Print and shaded views of the part. All mm, measured from the part's lowest x, y and z. Give positions to 0.01 mm unless a question says otherwise; leave off trailing zeros. Order: outer loops, then holes, each group sorted by start corner. A loop starts at its lowest first (then second) coordinate and runs counter-clockwise, first axis right, second up. Notation, with made-up numbers: (-4.75, -8) -> (13.25, -8) arc R17 cw to (13.25, 18) -> close; hole circle Ø7 at (68, -10). An arc over 180 degrees is marked (long way). One line per question, with ' | ' between items. Start each with the question number.
(1) Cut at A-A (z = 19.05). Give the cut face in (x, y), then the cut area to 3 significant figures.
(2) Drill centre lines: L1, parallel to X at y = 9.25, z = 31.75; L2, parallel to X at y = 1.75, z = 42.5; L3, parallel to Z at x = 45.72, y = 3. Where is each one in solid material? Low to high. Write a range as from..to.
(3) Cut at B-B (y = 6.5). Give the number of separate pieces and of enclosed holes in the cut face, then the cut area to 3 significant figures.
(4) Cut at C-C (x = 71.12). Give the cut face in (y, z), then the cut area to 3 significant figures.
(5) Pin check, flat tips, straight feed: pin 1 Ø2 at (y, z) = (9.5, 40) entering from -X; pin 2 Ø4 at (x, z) = (45.72, 31.75) entering from -Y; pin 3 Ø3 at (x, y) = (14.5, 2.5) entering from +Z; pin 4 Ø3 at (x, y) = (21, 4) entering from -Z. Stop position of each tip, or through.
(6) Cut at D-D (x = 13). Give the cut face in (y, z) (1 decimal).
(7) Pull direction X, two halves, no side cores. Call the marked faces 1, 2, 3 and 4: +X half, -X half, draft (parallel to the pull), parting line (faces both ways), or undercut.
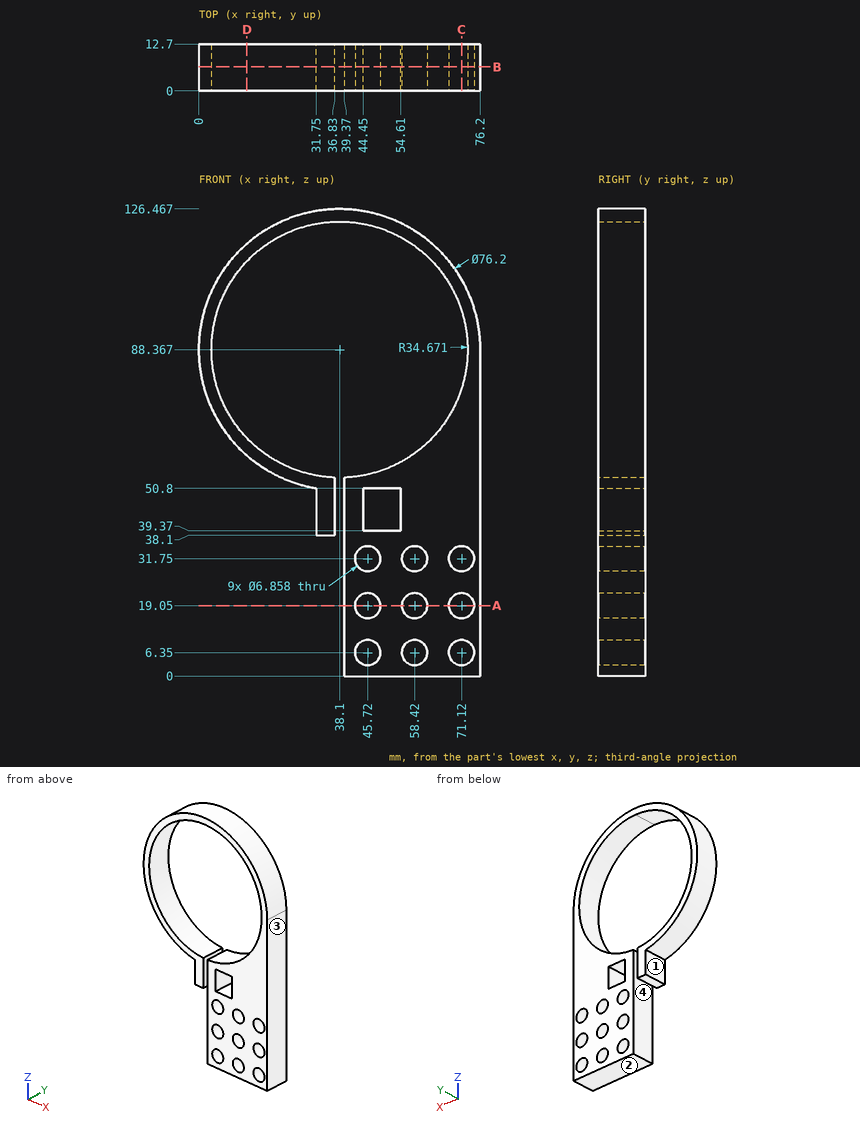
Result set:
1) outline: (39.37, 0) -> (42.29, 0) -> (42.29, 12.7) -> (39.37, 12.7) -> close; (49.15, 0) -> (54.99, 0) -> (54.99, 12.7) -> (49.15, 12.7) -> close; (61.85, 0) -> (67.69, 0) -> (67.69, 12.7) -> (61.85, 12.7) -> close; (74.55, 0) -> (76.2, 0) -> (76.2, 12.7) -> (74.55, 12.7) -> close | area: 206 mm2
2) L1: x = 39.37..42.29, 49.15..54.99, 61.85..67.69, 74.55..76.2 | L2: x = 31.75..36.83, 39.37..44.45, 54.61..76.2 | L3: z = 0..2.92, 9.78..15.62, 22.48..28.32, 35.18..39.37, 50.8..54.54, 122.19..125.7
3) separate pieces: 1 | enclosed holes: 10 | area: 2,550 mm2
4) outline: (0, 0) -> (12.7, 0) -> (12.7, 2.92) -> (0, 2.92) -> close; (0, 9.78) -> (12.7, 9.78) -> (12.7, 15.62) -> (0, 15.62) -> close; (0, 22.48) -> (12.7, 22.48) -> (12.7, 28.32) -> (0, 28.32) -> close; (0, 35.18) -> (12.7, 35.18) -> (12.7, 77.8) -> (0, 77.8) -> close; (0, 98.94) -> (12.7, 98.94) -> (12.7, 107.37) -> (0, 107.37) -> close | area: 834 mm2
5) pin 1: stops at x = 31.75 | pin 2: passes through | pin 3: stops at z = 119.4 | pin 4: stops at z = 53.61
6) outline: (0, 59.7) -> (12.7, 59.7) -> (12.7, 64.4) -> (0, 64.4) -> close; (0, 112.3) -> (12.7, 112.3) -> (12.7, 117) -> (0, 117) -> close
7) face 1: -X half | face 2: draft | face 3: +X half | face 4: undercut
